```python
from build123d import *

# Parameters (mm, degrees)
SKETCH1_R           = 3.175
SKETCH1_R_2         = 2.0828
SKETCH1_R_3         = 2
SKETCH1_R_4         = 2.413
SKETCH1_R_5         = 1.4224
SKETCH1_W           = 31.75
SKETCH1_H           = 9.525
BOSS_EXTRUDE1_DEPTH = 3.175


with BuildPart() as part:
    # Sketch1 → Boss-Extrude1 (new body)
    with BuildSketch(Plane.XY):
        Polygon((0, 0), (152.4, 0), (152.4, 177.8), (0, 177.8), (0, 123.19), (24.171108631, 123.19), (24.171108631, 97.79), (0, 97.79), align=None)
        with Locations((38.1, 82.55)):
            Circle(SKETCH1_R, mode=Mode.SUBTRACT)
        with Locations((63.5, 82.55)):
            Circle(SKETCH1_R, mode=Mode.SUBTRACT)
        with Locations((38.1, 57.15)):
            Circle(SKETCH1_R, mode=Mode.SUBTRACT)
        with Locations((63.5, 57.15)):
            Circle(SKETCH1_R, mode=Mode.SUBTRACT)
        with Locations((88.0237, 100.0125)):
            Circle(SKETCH1_R_2, mode=Mode.SUBTRACT)
        with Locations((100.7237, 100.0125)):
            Circle(SKETCH1_R_2, mode=Mode.SUBTRACT)
        with Locations((88.0237, 119.0625)):
            Circle(SKETCH1_R_2, mode=Mode.SUBTRACT)
        with Locations((100.7237, 119.0625)):
            Circle(SKETCH1_R_2, mode=Mode.SUBTRACT)
        with Locations((129.286, 109.5375)):
            Circle(SKETCH1_R, mode=Mode.SUBTRACT)
        with Locations((123.4, 139.48)):
            Circle(SKETCH1_R_3, mode=Mode.SUBTRACT)
        with Locations((147.4, 139.48)):
            Circle(SKETCH1_R_3, mode=Mode.SUBTRACT)
        with Locations((123.4, 157.48)):
            Circle(SKETCH1_R_3, mode=Mode.SUBTRACT)
        with Locations((147.4, 157.48)):
            Circle(SKETCH1_R_3, mode=Mode.SUBTRACT)
        with Locations((5, 6)):
            Circle(SKETCH1_R_3, mode=Mode.SUBTRACT)
        with Locations((29, 6)):
            Circle(SKETCH1_R_3, mode=Mode.SUBTRACT)
        with Locations((5, 24)):
            Circle(SKETCH1_R_3, mode=Mode.SUBTRACT)
        with Locations((29, 24)):
            Circle(SKETCH1_R_3, mode=Mode.SUBTRACT)
        with Locations((5, 139.48)):
            Circle(SKETCH1_R_3, mode=Mode.SUBTRACT)
        with Locations((29, 139.48)):
            Circle(SKETCH1_R_3, mode=Mode.SUBTRACT)
        with Locations((5, 157.48)):
            Circle(SKETCH1_R_3, mode=Mode.SUBTRACT)
        with Locations((29, 157.48)):
            Circle(SKETCH1_R_3, mode=Mode.SUBTRACT)
        with Locations((123.4, 6)):
            Circle(SKETCH1_R_3, mode=Mode.SUBTRACT)
        with Locations((147.4, 6)):
            Circle(SKETCH1_R_3, mode=Mode.SUBTRACT)
        with Locations((123.4, 24)):
            Circle(SKETCH1_R_3, mode=Mode.SUBTRACT)
        with Locations((147.4, 24)):
            Circle(SKETCH1_R_3, mode=Mode.SUBTRACT)
        with Locations((41.35, 155.575)):
            Circle(SKETCH1_R, mode=Mode.SUBTRACT)
        with Locations((41.35, 142.875)):
            Circle(SKETCH1_R, mode=Mode.SUBTRACT)
        with Locations((12.7, 57.15)):
            Circle(SKETCH1_R, mode=Mode.SUBTRACT)
        with Locations((12.7, 82.55)):
            Circle(SKETCH1_R, mode=Mode.SUBTRACT)
        with Locations((141.986, 109.5375)):
            Circle(SKETCH1_R, mode=Mode.SUBTRACT)
        with Locations((87.3125, 84.1375)):
            Circle(SKETCH1_R_4, mode=Mode.SUBTRACT)
        with Locations((87.3125, 134.9375)):
            Circle(SKETCH1_R_4, mode=Mode.SUBTRACT)
        with Locations((61.9125, 147.6375)):
            Circle(SKETCH1_R_5, mode=Mode.SUBTRACT)
        with Locations((112.7125, 147.6375)):
            Circle(SKETCH1_R_5, mode=Mode.SUBTRACT)
        with Locations((112.7125, 20.6375)):
            Circle(SKETCH1_R_5, mode=Mode.SUBTRACT)
        with Locations((61.9125, 20.6375)):
            Circle(SKETCH1_R_5, mode=Mode.SUBTRACT)
        with Locations((76.2, 28.575)):
            Circle(SKETCH1_R, mode=Mode.SUBTRACT)
        with Locations((76.2, 15.875)):
            Circle(SKETCH1_R, mode=Mode.SUBTRACT)
        with Locations((76.2, 165.1)):
            Circle(SKETCH1_R, mode=Mode.SUBTRACT)
        with Locations((76.2, 152.4)):
            Circle(SKETCH1_R, mode=Mode.SUBTRACT)
        with Locations((85.725, 109.5375)):
            Rectangle(SKETCH1_W, SKETCH1_H, mode=Mode.SUBTRACT)
    extrude(amount=BOSS_EXTRUDE1_DEPTH)


solid = part.part
```
Input: part model. Units: mm. Frame: model coordinates. Coordinates: 2 decimals unless noted, no trailing zeros. Loops run counter-clockwise (first coordinate to the right, second up) from the corner with the lowest first, then second, coordinate; pieces in that order, holes last.
Q1. Mould query, pull axis Y, two halves, no side actions, for faces 1 (the flat face through (75, 90, 0)), 2 (the cylindrical face through (30.908, 6.601, 1.565)). Classes: +Y half, -Y half, draft (parallel to the pull), parting line (faces both ways), or undercut.
Results are:
face 1: draft
face 2: undercut
Q2. Section C-C, the plane y = 6. Return the cut outline in (x, z) (3 decimals).
Results are:
outline: (0, 0) - (3, 0) - (3, 3.175) - (0, 3.175) - close; (7, 0) - (27, 0) - (27, 3.175) - (7, 3.175) - close; (31, 0) - (121.4, 0) - (121.4, 3.175) - (31, 3.175) - close; (125.4, 0) - (145.4, 0) - (145.4, 3.175) - (125.4, 3.175) - close; (149.4, 0) - (152.4, 0) - (152.4, 3.175) - (149.4, 3.175) - close
Q3. Section D-D, the plane x = 5. Return the cut outline in (y, z) (3 decimals), and give its area (3 significant figures).
Results are:
outline: (0, 0) - (4, 0) - (4, 3.175) - (0, 3.175) - close; (8, 0) - (22, 0) - (22, 3.175) - (8, 3.175) - close; (26, 0) - (97.79, 0) - (97.79, 3.175) - (26, 3.175) - close; (123.19, 0) - (137.48, 0) - (137.48, 3.175) - (123.19, 3.175) - close; (141.48, 0) - (155.48, 0) - (155.48, 3.175) - (141.48, 3.175) - close; (159.48, 0) - (177.8, 0) - (177.8, 3.175) - (159.48, 3.175) - close
area: 433 mm2
Q4. Section A-A, the plane x = 96.5. Return the cut outline in (y, z) (3 decimals).
Results are:
outline: (0, 0) - (104.775, 0) - (104.775, 3.175) - (0, 3.175) - close; (114.3, 0) - (177.8, 0) - (177.8, 3.175) - (114.3, 3.175) - close
Q5. Line query: line 1 along X through (y, z) = (139.5, 0.65); line 2 along Y through (x, z) = (76.2, 1.7) (3 decimals); line 3 along Y through (x, z) = (123, 1.5). Output: solid intervals per line, ascending.
Results are:
line 1: x = 0 to 3, 7 to 27, 31 to 121.4, 125.4 to 145.4, 149.4 to 152.4
line 2: y = 0 to 12.7, 19.05 to 25.4, 31.75 to 104.775, 114.3 to 149.225, 155.575 to 161.925, 168.275 to 177.8
line 3: y = 0 to 4.04, 7.96 to 22.04, 25.96 to 137.52, 141.44 to 155.52, 159.44 to 177.8
Q6. Section B-B, the plane y = 165.1. Return the cut outline in (x, z) (3 decimals).
Results are:
outline: (0, 0) - (73.025, 0) - (73.025, 3.175) - (0, 3.175) - close; (79.375, 0) - (152.4, 0) - (152.4, 3.175) - (79.375, 3.175) - close
